Can you work these out from the model? Positions are in its coordinate system, mm. A direction names the side the tool comes from. Coordinates: 2 decimals unless noted, no trailing zeros. Write each loop counter-clockwise with the first axis right and the second up, starting at its lowest first coordinate (ties: lowest second). Pieces come first, ordered by that corner, then holes. Notation, with made-up numbers: (27.25, 19) -> (75.25, 19) arc R35 cw to (75.25, 53) -> close; hole circle Ø1 at (31, 4). An arc over 180 degrees is marked (long way). Use one line per item in the form item = value.
```python
from build123d import *

# Parameters (mm, degrees)
SKETCH1_R           = 7.4803
BOSS_EXTRUDE1_DEPTH = 5.8928
SKETCH2_R           = 2.7813
CUT_EXTRUDE1_DEPTH  = 3.3782
BOSS_EXTRUDE2_DEPTH = 3.8354
BOSS_EXTRUDE3_DEPTH = 2.0574
SKETCH6_R           = 4.1656
CUT_EXTRUDE2_DEPTH  = 0.9398
SKETCH7_R           = 1.6002
SKETCH7_R_2         = 1.27
SKETCH7_W           = 18.255027212
SKETCH7_H           = 1.143
CUT_EXTRUDE3_DEPTH  = 6.8928


with BuildPart() as part:
    # Sketch1 → Boss-Extrude1 (new body)
    with BuildSketch(Plane(origin=(0, 0, 0), x_dir=(1, 0, 0), z_dir=(0, 1, 0))):
        Circle(SKETCH1_R)
    extrude(amount=BOSS_EXTRUDE1_DEPTH)

    # Sketch2 → Cut-Extrude1 (cut)
    with BuildSketch(Plane.XZ):
        Circle(SKETCH2_R)
    extrude(amount=-CUT_EXTRUDE1_DEPTH, mode=Mode.SUBTRACT)

    # Sketch4 → Boss-Extrude2 (add)
    with BuildSketch(Plane(origin=(0, 5.8928, 0), x_dir=(1, 0, 0), z_dir=(0, 1, 0))):
        with BuildLine():
            Line((-24.0919, 3.7338), (-6.481791855, 3.7338))
            ThreePointArc((-6.481791855, 3.7338), (-7.4803, 0), (-6.481791855, -3.7338))
            Line((-6.481791855, -3.7338), (-24.0919, -3.7338))
            ThreePointArc((-24.0919, -3.7338), (-27.8257, 0), (-24.0919, 3.7338))
        make_face()
    extrude(amount=-BOSS_EXTRUDE2_DEPTH)

    # Sketch5 → Boss-Extrude3 (add)
    with BuildSketch(Plane.XZ.offset(-2.0574)):
        with BuildLine():
            Line((-24.0284, 3.0099), (-19.9644, 3.0099))
            ThreePointArc((-19.9644, 3.0099), (-16.9545, 0), (-19.9644, -3.0099))
            Line((-19.9644, -3.0099), (-24.0284, -3.0099))
            ThreePointArc((-24.0284, -3.0099), (-27.0383, 0), (-24.0284, 3.0099))
        make_face()
    extrude(amount=BOSS_EXTRUDE3_DEPTH)

    # Sketch6 → Cut-Extrude2 (cut)
    with BuildSketch(Plane(origin=(0, 5.8928, 0), x_dir=(1, 0, 0), z_dir=(0, 1, 0))):
        Circle(SKETCH6_R)
    extrude(amount=-CUT_EXTRUDE2_DEPTH, mode=Mode.SUBTRACT)

    # Sketch7 → Cut-Extrude3 (cut, through all)
    with BuildSketch(Plane(origin=(0, 5.8928, 0), x_dir=(1, 0, 0), z_dir=(0, 1, 0))):
        with Locations((-9.0297, 0)):
            Circle(SKETCH7_R)
        Circle(SKETCH7_R)
        with Locations((-24.0157, 0)):
            Circle(SKETCH7_R_2)
        with Locations((-19.9009, 0)):
            Circle(SKETCH7_R_2)
        with Locations((0.097813606, 0)):
            Rectangle(SKETCH7_W, SKETCH7_H)
    extrude(amount=-CUT_EXTRUDE3_DEPTH, mode=Mode.SUBTRACT)


solid = part.part
```
Q1. If I drill on line 1 (Z direction, x = -24, y = 4.5); line 2 (X direction, y = 0.7, z = -0.25); line 3 (Z direction, x = -7, y = 5.2), over which ranges is the centre line in solid material (lowest first)? Write a range as from..to.
Return value:
line_1 = -3.73..-1.27, 1.27..3.73
line_2 = -27.03..-25.26, -22.77..-21.15, -18.66..-16.96
line_3 = -3.73..-0.57, 0.57..3.73
Q2. Will these pins go through, and if not, where does the flat tip stop? pin 1 (0.6 mm diameter, centred on x = -21.5, y = 1, fed in from -Z); pin 2 (1.8 mm diameter, centred on x = 4.5, y = 3, fed in from +Z); pin 3 (1.8 mm diameter, centred on x = -5.5, y = 3, fed in from +Z).
Return value:
pin_1 = -3.01
pin_2 = 6.56
pin_3 = 5.9
Q3. Suppose I cut it at A-A (y = 0.85). Write out the boundary of the cut face in (x, z), then the cut area to 3 significant figures.
Return value:
outline = (-24.03, -3.01) -> (-19.96, -3.01) arc R3.01 ccw to (-19.96, 3.01) -> (-24.03, 3.01) arc R3.01 ccw to start; (-7.46, -0.57) arc R7.48 ccw to (7.46, -0.57) -> (2.72, -0.57) arc R2.78 cw to (-2.72, -0.57) -> close; (-7.46, 0.57) -> (-2.72, 0.57) arc R2.78 cw to (2.72, 0.57) -> (7.46, 0.57) arc R7.48 ccw to start; hole circle Ø2.54 at (-24.02, 0); hole circle Ø2.54 at (-19.9, 0)
area = 184 mm2
Q4. Suppose I cut it at D-D (x = -19). Write out the boundary of the cut face in (y, z), then the cut area to 3 significant figures.
Return value:
outline = (0, -2.85) -> (2.06, -2.85) -> (2.06, -3.73) -> (5.89, -3.73) -> (5.89, -0.9) -> (0, -0.9) -> close; (0, 0.9) -> (5.89, 0.9) -> (5.89, 3.73) -> (2.06, 3.73) -> (2.06, 2.85) -> (0, 2.85) -> close
area = 29.8 mm2
Q5. Suppose I cut it at B-B (z = 0). Write out the boundary of the cut face in (x, y), then the cut area to 3 significant figures.
Return value:
outline = (-27.83, 2.06) -> (-27.04, 2.06) -> (-27.04, 0) -> (-25.29, 0) -> (-25.29, 5.89) -> (-27.83, 5.89) -> close; (-22.75, 0) -> (-21.17, 0) -> (-21.17, 5.89) -> (-22.75, 5.89) -> close; (-18.63, 0) -> (-16.95, 0) -> (-16.95, 2.06) -> (-10.63, 2.06) -> (-10.63, 5.89) -> (-18.63, 5.89) -> close
area = 56.8 mm2
Q6. For faces 1 (the flat face through (-15, 4, -3.734)), 2 (the flat face through (-5, 3, -0.572)), 3 (the cylindrical face through (0, 4.2, -1.6)), 4 (the flat face through (-22, 1, 3.01)), which set-ups out of +Z, -Z, +X, -X, +Y, -Y let a thin tool reach every point of the face, with its end or its side?
Return value:
face_1 = -Z, -X, +Y, -Y
face_2 = +X, +Y, -Y
face_3 = +Y, -Y
face_4 = +Z, -X, -Y
Q7. Suppose I cut it at C-C (y = 3.7). Write out the boundary of the cut face in (x, z).
Return value:
outline = (-24.09, -3.73) -> (-6.48, -3.73) arc R7.48 ccw to (7.46, -0.57) -> (1.49, -0.57) arc R1.6 cw to (-1.49, -0.57) -> (-7.54, -0.57) arc R1.6 cw (long way) to (-7.54, 0.57) -> (-1.49, 0.57) arc R1.6 cw to (1.49, 0.57) -> (7.46, 0.57) arc R7.48 ccw to (-6.48, 3.73) -> (-24.09, 3.73) arc R3.73 ccw to start; hole circle Ø2.54 at (-24.02, 0); hole circle Ø2.54 at (-19.9, 0)
